Work out the finished part from the listing and answer in its coordinate system (mm). Round coordinates to 2 decimals unless told otherwise and drop trailing zeros. Loops run counter-clockwise (first coordinate to the right, second up) from the corner with the lowest first, then second, coordinate; pieces in that order, holes last. Notation, with made-up numbers: (-20.5, -23.75) - (-9.5, -23.75) arc R20 cw to (-9.5, 11.25) - close; hole circle Ø2 at (-19, 43.25). An arc over 180 degrees is marked (long way). Return JSON: item names as keys, results as strings.
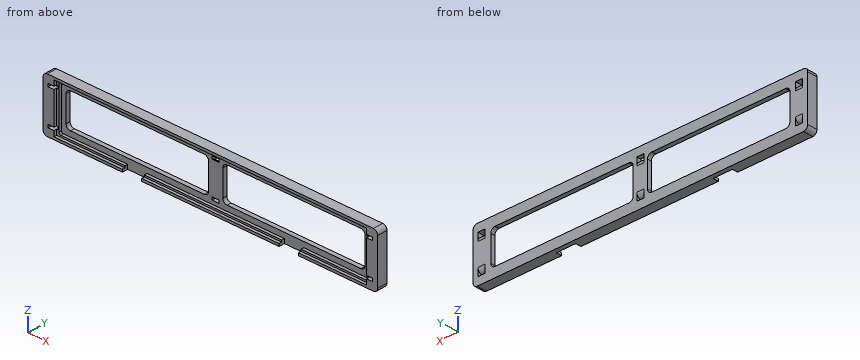
from build123d import *

# Parameters (mm, degrees)
F0_W        = 5
F0_H        = 2
F1_DEPTH    = 3
F2_W        = 5
F2_H        = 2
F3_DEPTH    = 4
F4_W        = 219.5
F4_H        = 34
F4_W_2      = 214.53166008
F4_H_2      = 28.9933998138
F5_DEPTH    = 2
F6_W        = 13.5
F6_H        = 4
F7_DEPTH    = 25
F8_T1_DEPTH = 5
F8_T3_DEPTH = 5
F8_T5_DEPTH = 5


# Not quite as in the source:
# - a fillet or chamfer that OpenCascade refuses, or shapes differently, is made with other operations: its cross-section is extruded or revolved along the edge and cut away or added
# - a feature names something its author has since deleted; it is built from what else it names


with BuildPart() as f1:
    # F0 (on Front) → F1 (new body)
    with BuildSketch(Plane.XZ):
        with BuildLine():
            ThreePointArc((117.5, 15.75), (116.6213203436, 17.8713203436), (114.5, 18.75))
            Line((114.5, 18.75), (-114.5, 18.75))
            ThreePointArc((-114.5, 18.75), (-116.6213203436, 17.8713203436), (-117.5, 15.75))
            Line((-117.5, 15.75), (-117.5, -15.75))
            ThreePointArc((-117.5, -15.75), (-116.6213203436, -17.8713203436), (-114.5, -18.75))
            Line((-114.5, -18.75), (114.5, -18.75))
            ThreePointArc((114.5, -18.75), (116.6213203436, -17.8713203436), (117.5, -15.75))
            Line((117.5, -15.75), (117.5, 15.75))
        make_face()
        with Locations((-111.5, -12.25)):
            Rectangle(F0_W, F0_H, mode=Mode.SUBTRACT)
        with Locations((0, -12.25)):
            Rectangle(F0_W, F0_H, mode=Mode.SUBTRACT)
        with Locations((111.5, -12.25)):
            Rectangle(F0_W, F0_H, mode=Mode.SUBTRACT)
        with BuildLine():
            Line((-102, 12), (-8, 12))
            ThreePointArc((-8, 12), (-5.8786796564, 11.1213203436), (-5, 9))
            Line((-5, 9), (-5, -9))
            ThreePointArc((-5, -9), (-5.8786796564, -11.1213203436), (-8, -12))
            Line((-8, -12), (-102, -12))
            ThreePointArc((-102, -12), (-104.1213203436, -11.1213203436), (-105, -9))
            Line((-105, -9), (-105, 9))
            ThreePointArc((-105, 9), (-104.1213203436, 11.1213203436), (-102, 12))
        make_face(mode=Mode.SUBTRACT)
        with Locations((-111.5, 12.25)):
            Rectangle(F0_W, F0_H, mode=Mode.SUBTRACT)
        with BuildLine():
            Line((8, 12), (102, 12))
            ThreePointArc((102, 12), (104.1213203436, 11.1213203436), (105, 9))
            Line((105, 9), (105, -9))
            ThreePointArc((105, -9), (104.1213203436, -11.1213203436), (102, -12))
            Line((102, -12), (8, -12))
            ThreePointArc((8, -12), (5.8786796564, -11.1213203436), (5, -9))
            Line((5, -9), (5, 9))
            ThreePointArc((5, 9), (5.8786796564, 11.1213203436), (8, 12))
        make_face(mode=Mode.SUBTRACT)
        with Locations((0, 12.25)):
            Rectangle(F0_W, F0_H, mode=Mode.SUBTRACT)
        with Locations((111.5, 12.25)):
            Rectangle(F0_W, F0_H, mode=Mode.SUBTRACT)
    extrude(amount=F1_DEPTH)

    # F2 (on face) → F3 (join)
    with BuildSketch(Plane.XZ.offset(3)):
        with BuildLine():
            Line((-114.5, -18.75), (114.5, -18.75))
            ThreePointArc((114.5, -18.75), (116.6213203436, -17.8713203436), (117.5, -15.75))
            Line((117.5, -15.75), (117.5, 15.75))
            ThreePointArc((117.5, 15.75), (116.6213203436, 17.8713203436), (114.5, 18.75))
            Line((114.5, 18.75), (-114.5, 18.75))
            ThreePointArc((-114.5, 18.75), (-116.6213203436, 17.8713203436), (-117.5, 15.75))
            Line((-117.5, 15.75), (-117.5, -15.75))
            ThreePointArc((-117.5, -15.75), (-116.6213203436, -17.8713203436), (-114.5, -18.75))
        make_face()
        with Locations((-111.5, -12.25)):
            Rectangle(F2_W, F2_H, mode=Mode.SUBTRACT)
        with Locations((111.5, -12.25)):
            Rectangle(F2_W, F2_H, mode=Mode.SUBTRACT)
        with BuildLine():
            Line((-107.25, 15.75), (107.25, 15.75))
            ThreePointArc((107.25, 15.75), (107.9571067812, 15.4571067812), (108.25, 14.75))
            Line((108.25, 14.75), (108.25, -14.75))
            ThreePointArc((108.25, -14.75), (107.9571067812, -15.4571067812), (107.25, -15.75))
            Line((107.25, -15.75), (-107.25, -15.75))
            ThreePointArc((-107.25, -15.75), (-107.9571067812, -15.4571067812), (-108.25, -14.75))
            Line((-108.25, -14.75), (-108.25, 14.75))
            ThreePointArc((-108.25, 14.75), (-107.9571067812, 15.4571067812), (-107.25, 15.75))
        make_face(mode=Mode.SUBTRACT)
        with Locations((-111.5, 12.25)):
            Rectangle(F2_W, F2_H, mode=Mode.SUBTRACT)
        with Locations((111.5, 12.25)):
            Rectangle(F2_W, F2_H, mode=Mode.SUBTRACT)
    extrude(amount=F3_DEPTH)

    # F4 (on face) → F5 (cut)
    with BuildSketch(Plane.XZ.offset(7)):
        Rectangle(F4_W, F4_H)
        Rectangle(F4_W_2, F4_H_2, mode=Mode.SUBTRACT)
    extrude(amount=-F5_DEPTH, mode=Mode.SUBTRACT)

    # F6 (on face) → F7 (cut)
    with BuildSketch(Plane(origin=(0, 0, -18.75), x_dir=(1, 0, 0), z_dir=(0, 0, -1))):
        with Locations((-55, 5)):
            Rectangle(F6_W, F6_H)
        with Locations((55, 5)):
            Rectangle(F6_W, F6_H)
    extrude(amount=-F7_DEPTH, mode=Mode.SUBTRACT)

    # F8: fillet of radius 3.5 on 6 edges, made by hand

    # F8_s2 → F8_t1 (cut)
    with BuildSketch(Plane.YZ.offset(-2.5)):
        with BuildLine():
            ThreePointArc((0, 7.7858983849), (-0.8542486889, 10.0771862323), (-3, 11.25))
            Line((-3, 11.25), (0, 11.25))
            Line((0, 11.25), (0, 7.7858983849))
        make_face()
        with BuildLine():
            ThreePointArc((0, -7.7858983849), (-0.8542486889, -10.0771862323), (-3, -11.25))
            Line((-3, -11.25), (0, -11.25))
            Line((0, -11.25), (0, -7.7858983849))
        make_face()
    extrude(amount=F8_T1_DEPTH, mode=Mode.SUBTRACT)

    # F8_s4 → F8_t3 (cut)
    with BuildSketch(Plane.YZ.offset(109)):
        with BuildLine():
            ThreePointArc((0, 7.75), (-1.0251262658, 10.2248737342), (-3.5, 11.25))
            Line((-3.5, 11.25), (0, 11.25))
            Line((0, 11.25), (0, 7.75))
        make_face()
        with BuildLine():
            ThreePointArc((0, -7.75), (-1.0251262658, -10.2248737342), (-3.5, -11.25))
            Line((-3.5, -11.25), (0, -11.25))
            Line((0, -11.25), (0, -7.75))
        make_face()
    extrude(amount=F8_T3_DEPTH, mode=Mode.SUBTRACT)

    # F8_s6 → F8_t5 (cut)
    with BuildSketch(Plane.YZ.offset(-114)):
        with BuildLine():
            ThreePointArc((0, -7.75), (-1.0251262658, -10.2248737342), (-3.5, -11.25))
            Line((-3.5, -11.25), (0, -11.25))
            Line((0, -11.25), (0, -7.75))
        make_face()
        with BuildLine():
            ThreePointArc((0, 7.75), (-1.0251262658, 10.2248737342), (-3.5, 11.25))
            Line((-3.5, 11.25), (0, 11.25))
            Line((0, 11.25), (0, 7.75))
        make_face()
    extrude(amount=F8_T5_DEPTH, mode=Mode.SUBTRACT)


solid = f1.part
1) Section B-B (x = 16) is taken. Give the vertices of the cut face in (y, z), and give its area (3 significant figures).
Verdict:
{"outline": "(-7, -18.75) - (0, -18.75) - (0, -12) - (-3, -12) - (-3, -15.75) - (-5, -15.75) - (-5, -17) - (-7, -17) - close; (-7, 17) - (-5, 17) - (-5, 15.75) - (-3, 15.75) - (-3, 12) - (0, 12) - (0, 18.75) - (-7, 18.75) - close", "area": "59.5 mm2"}
2) Find the intervals of material crossed by L1, parallel to X at y = -3.75, z = -16; L2, parallel to X at y = -0.25, z = -4; L3, parallel to Z at x = -47, y = -0.75, in increasing order.
Verdict:
{"L1": "x = -117.49 to -61.75, -48.25 to 48.25, 61.75 to 117.49", "L2": "x = -117.5 to -105, -5 to 5, 105 to 117.5", "L3": "z = -18.75 to -12, 12 to 18.75"}
3) Flat-ended cylindrical pins translate along their axes: pin 1 (3.5 mm diameter, centred on y = -5, z = -17, fed in from +X); pin 2 (0.6 mm diameter, centred on x = 14.5, z = -16, fed in from -Y). Find the tip coordinate at first contact, or state that the pin passes through.
Verdict:
{"pin 1": "stops at x = 117.5", "pin 2": "stops at y = -5"}
4) Section A-A (z = 0) is taken. Give the vertices of the cut face in (x, y), and give its area (3 significant figures).
Verdict:
{"outline": "(-117.5, -7) - (-109.75, -7) - (-109.75, -5) - (-108.25, -5) - (-108.25, -3) - (-105, -3) - (-105, 0) - (-117.5, 0) - close; (-5, -3) - (5, -3) - (5, 0) - (-5, 0) - close; (105, -3) - (108.25, -3) - (108.25, -5) - (109.75, -5) - (109.75, -7) - (117.5, -7) - (117.5, 0) - (105, 0) - close", "area": "173 mm2"}
5) Section C-C (y = -1.5) is taken. Count the separate pieces of the cut face and the enclosed holes in it, and give its area (3 significant figures).
Verdict:
{"separate pieces": "1", "enclosed holes": "8", "area": "3,940 mm2"}
